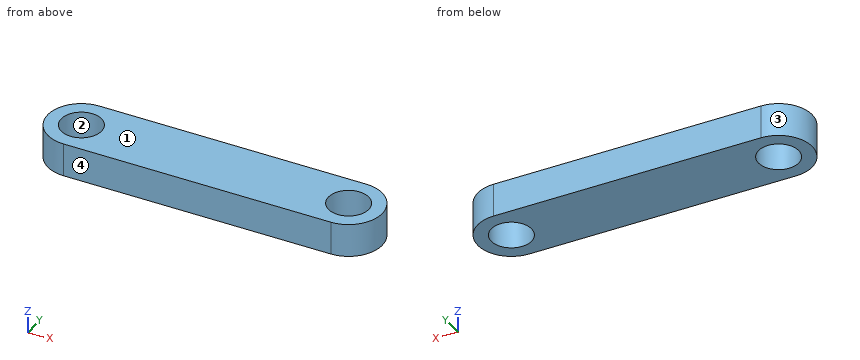
from build123d import *

# Parameters (mm, degrees)
SKETCH1_R           = 3
BOSS_EXTRUDE1_DEPTH = 5
SKETCH2_R           = 3
CUT_EXTRUDE2_DEPTH  = 15


with BuildPart() as part:
    # Sketch1 → Boss-Extrude1 (new body)
    with BuildSketch(Plane.XY):
        with BuildLine():
            Line((19.65, -5), (-19.65, -5))
            ThreePointArc((-19.65, -5), (-24.65, 0), (-19.65, 5))
            Line((-19.65, 5), (19.65, 5))
            ThreePointArc((19.65, 5), (24.65, 0), (19.65, -5))
        make_face()
        with Locations((-19.65, 0)):
            Circle(SKETCH1_R, mode=Mode.SUBTRACT)
    extrude(amount=BOSS_EXTRUDE1_DEPTH)

    # Sketch2 → Cut-Extrude2 (cut)
    with BuildSketch(Plane(origin=(0, 0, 0), x_dir=(-1, 0, 0), z_dir=(0, 0, -1))):
        with Locations((-19.65, 0)):
            Circle(SKETCH2_R)
    extrude(amount=-CUT_EXTRUDE2_DEPTH, mode=Mode.SUBTRACT)


solid = part.part
Build history of the part. All positions in model axes, mm. Face numbers are marked on the shaded views. Coordinates: 2 decimals unless noted, no trailing zeros. Order: outer loops, then holes, each group sorted by start corner. A loop starts at its lowest first (then second) coordinate and runs counter-clockwise, first axis right, second up. Notation, with made-up numbers: (49.25, 87.5) - (108.25, 87.5) arc R23 ccw to (108.25, 113.5) - close; hole circle Ø10 at (78, 4). An arc over 180 degrees is marked (long way). Write each question's results on one line, items separated by ' | '. Start each with the question number.
Item 1: Band-saw the part on C-C on y = 2. Write the cut outline in (x, z), and give its area (3 significant figures).
Item 2: Wall check: probe 1 along Y at (x, z) = (19.65, 3.5); probe 2 along X at (y, z) = (-0.5, 3.15); probe 3 along X at (y, z) = (2, 0.7). Give the ranges that are in metal, low to high. Write a range as [from, to].
Item 3: Mould opens along Y. For the marked faces 1, 2, 3 and 4 say: released by +Y, released by -Y, zero draft, split by the parting line, or undercut.
Item 4: Band-saw the part on B-B on z = 3.05. Write the cut outline in (x, y).
Item 5: Flat gauge pins, fed straight in: pin 1 (2 mm diameter, centred on y = 0.5, z = 4.5, fed in from +X); pin 2 (1 mm diameter, centred on y = 1, z = 3, fed in from -X); pin 3 (5.5 mm diameter, centred on x = -19.65, y = 0, fed in from -Z). Where does each tip first touch, or does it go through?
Item 6: Band-saw the part on A-A on y = -2.25. Write the cut outline in (x, z).
Numbers:
1) outline: (-24.23, 0) - (-21.89, 0) - (-21.89, 5) - (-24.23, 5) - close; (-17.41, 0) - (17.41, 0) - (17.41, 5) - (-17.41, 5) - close; (21.89, 0) - (24.23, 0) - (24.23, 5) - (21.89, 5) - close | area: 198 mm^2
2) probe 1: [-5, -3], [3, 5] | probe 2: [-24.62, -22.61], [-16.69, 16.69], [22.61, 24.62] | probe 3: [-24.23, -21.89], [-17.41, 17.41], [21.89, 24.23]
3) face 1: zero draft | face 2: undercut | face 3: split by the parting line | face 4: released by -Y
4) outline: (-19.65, -5) - (19.65, -5) arc R5 ccw to (19.65, 5) - (-19.65, 5) arc R5 ccw to start; hole circle Ø6 at (-19.65, 0); hole circle Ø6 at (19.65, 0)
5) pin 1: x = 24.65 | pin 2: x = -24.62 | pin 3: through
6) outline: (-24.12, 0) - (-21.63, 0) - (-21.63, 5) - (-24.12, 5) - close; (-17.67, 0) - (17.67, 0) - (17.67, 5) - (-17.67, 5) - close; (21.63, 0) - (24.12, 0) - (24.12, 5) - (21.63, 5) - close
